Input: dimensioned drawing with shaded views. Units: mm. Origin: part minimum x, y, z. A direction names the side the tool comes from. Round coordinates to 2 decimals unless told otherwise and drop trailing zeros. Loops run counter-clockwise (first coordinate to the right, second up) from the corner with the lowest first, then second, coordinate; pieces in that order, holes last.
Item 1: Section query C-C on z = 6.25. Return loops of the section in (x, y), then the cut area to 3 significant figures.
Item 2: Section query A-A on y = 80. Return loops of the section in (x, z), then the cut area to 3 significant figures.
Item 3: Section query D-D on y = 28.5. Return loops of the section in (x, z), then the cut area to 3 significant figures.
Item 4: First-contact query: P1, Ø1, axis at x = 78, z = 11.5, coming from the +Y side; P2, Ø8, axis at x = 92.5, y = 117, coming from the +Z side; P3, Ø3, axis at x = 90.5, z = 8.5, coming from the +Y side. Flat tips, straight axial feed; report the tip coordinate or a pass-through.
Item 5: Access query for the marked faces 1 and 2. Directions: +Z, -Z, +X, -X, +Y, -Y. A direction counts if a zero-diameter tool reaches every point of the face in a straight line with its end or side. Return the directions, or none.
Item 6: Ray query, L1, parallel to Y at x = 80, z = 8; L2, parallel to Z at x = 72.5, y = 99.5; L3, parallel to X at y = 83, z = 9.25. Return the intervals inside material, ascending.
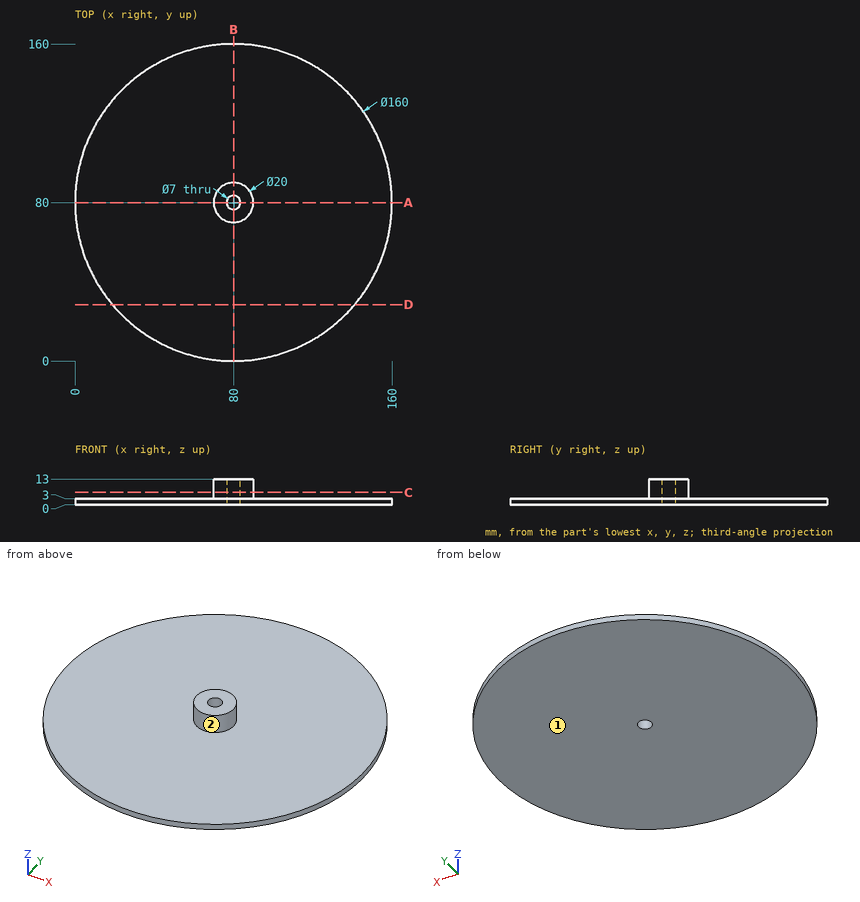
Data:
1. outline: circle Ø20 at (80, 80); hole circle Ø7 at (80, 80)
1. area: 276 mm2
2. outline: (0, 0) - (76.5, 0) - (76.5, 13) - (70, 13) - (70, 3) - (0, 3) - close; (83.5, 0) - (160, 0) - (160, 3) - (90, 3) - (90, 13) - (83.5, 13) - close
2. area: 589 mm2
3. outline: (18.78, 0) - (141.22, 0) - (141.22, 3) - (18.78, 3) - close
3. area: 367 mm2
4. P1: stops at y = 89.89
4. P2: stops at z = 3
4. P3: stops at y = 84.36
5. face 1: -Z, +X, -X, +Y, -Y
5. face 2: +Z
6. L1: y = 70 to 76.5, 83.5 to 90
6. L2: z = 0 to 3
6. L3: x = 70.46 to 78.2, 81.8 to 89.54
